from build123d import *

# Parameters (mm, degrees)
F0_W     = 3.81
F0_H     = 12.7
F1_DEPTH = 12.7
F3_DEPTH = 4.445
F4_W     = 3.81
F4_H     = 12.7
F5_DEPTH = 12.7
F6_R     = 1.61925
F7_DEPTH = 25.4


with BuildPart() as f1:
    # F0 (on Front) → F1 (new body)
    with BuildSketch(Plane.XZ):
        Rectangle(F0_W, F0_H)
    extrude(amount=F1_DEPTH)

    # F2 (on face) → F3 (join, symmetric)
    with BuildSketch(Plane(origin=(0, 0, 0), x_dir=(-1, 0, 0), z_dir=(0, 1, 0))):
        Polygon((-1.905, 6.35), (-1.905, -6.35), (1.905, -6.35), (1.905, -2.54), (1.905, 6.35), align=None)
        with BuildLine():
            Line((1.905, -6.35), (-1.905, -6.35))
            ThreePointArc((-1.905, -6.35), (4.5990768363, -9.0440768363), (1.905, -2.54))
            Line((1.905, -2.54), (1.905, -6.35))
        make_face()
    extrude(amount=F3_DEPTH, both=True)

    # F4 (on face) → F5 (join)
    with BuildSketch(Plane(origin=(0, 0, 0), x_dir=(-1, 0, 0), z_dir=(0, 1, 0))):
        Rectangle(F4_W, F4_H)
    extrude(amount=F5_DEPTH)

    # F6 (on face) → F7 (cut)
    with BuildSketch(Plane(origin=(0, 12.7, 0), x_dir=(-1, 0, 0), z_dir=(0, 1, 0))):
        with Locations((1.905, -6.35)):
            Circle(F6_R)
    extrude(amount=-F7_DEPTH, mode=Mode.SUBTRACT)


solid = f1.part
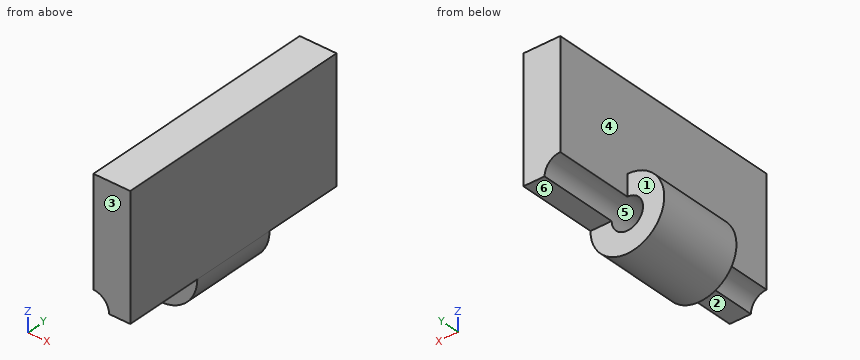
For this review, take the finished solid that the model builds, in its own axes (mm). Face numbers are marked on the shaded views. A direction names the side the tool comes from. Coordinates: 2 decimals unless noted, no trailing zeros. Loops run counter-clockwise (first coordinate to the right, second up) from the corner with the lowest first, then second, coordinate; pieces in that order, holes last. Notation, with made-up numbers: (-34, -16) -> (-13, -16) arc R17 cw to (-13, 13) -> close; hole circle Ø3 at (67, 75.5). An arc over 180 degrees is marked (long way). Write each question's results on one line, items separated by ' | '.
Q1. Add section C-C, the plane x = -1. State the section outline as (y, z) points (3 decimals), then the cut area to 3 significant figures.
Taken from the geometry:
outline: (-12.7, -5.007) -> (12.7, -5.007) -> (12.7, 6.35) -> (-12.7, 6.35) -> close; (-4.445, -10.051) -> (4.445, -10.051) -> (4.445, -7.693) -> (-4.445, -7.693) -> close | area: 309 mm²
Q2. Mouldability with a two-part tool opening along X and no side actions: class the marked faces 4, 5 and 6 as +X half, -X half, draft (parallel to the pull), parting line (faces both ways), or undercut.
Taken from the geometry:
face 4: -X half | face 5: undercut | face 6: draft
Q3. To check wall thickness, follow line 1 along X through (y, z) = (2.5, -6.35) (3 decimals); line 2 along Z through (x, y) = (0.5, -11); line 3 along Z through (x, y) = (-2.5, -4.25). State the ranges of each line that lie inside material, in increasing order. Write a range as [from, to].
Taken from the geometry:
line 1: [-5.715, -3.524], [-0.286, 1.905] | line 2: [-6.35, 6.35] | line 3: [-10.11, -7.86], [-4.84, -2.59]
Q4. For pin 1 Ø5.5 at (y, z) = (2.5, 2) entering from -X (3 decimals); pin 2 Ø1.8 at (x, y) = (0.5, -8.5) entering from -Z; pin 3 Ø3 at (x, z) = (-4.5, -2) entering from +Y (3 decimals), all flat-tipped, find the tip position at first contact; note any pin that passes through.
Taken from the geometry:
pin 1: x = -1.905 | pin 2: z = -6.35 | pin 3: y = 4.445
Q5. Add section B-B, the plane z = -6. State the section outline as (x, y) points (3 decimals).
Taken from the geometry:
outline: (-5.699, -4.445) -> (-3.486, -4.445) -> (-3.486, 4.445) -> (-5.699, 4.445) -> close; (-0.324, -12.7) -> (1.905, -12.7) -> (1.905, 12.7) -> (-0.324, 12.7) -> close
Q6. Machinability: for the marked faces 1, 2 and 3, which of the approach directions +Z, -Z, +X, -X, +Y, -Y give a long, thin tool a straight path to every point of the face, cutting with its end or side? Answer none if there is none.
Taken from the geometry:
face 1: -Z, -X, +Y | face 2: -Z, +X, -X, -Y | face 3: +Z, -Z, +X, -X, -Y
